Drawing for the job (mm, zero at the part's lowest x, y, z). A direction names the side the tool comes from. Give positions to 0.01 mm unless a question says otherwise; leave off trailing zeros. Loops run counter-clockwise (first coordinate to the right, second up) from the corner with the lowest first, then second, coordinate; pieces in that order, holes last.
1) Band-saw the part on B-B on x = 5. List the corners of the cut face in (y, z).
2) Two-plate mould, pull along Y, no slides. Class the marked faces 1, 2 and 3: +Y half, -Y half, draft (parallel to the pull), parting line (faces both ways), or undercut.
3) 3-axis set-ups, long thin cutter, end or side, ignore diameter. For the marked faces 4 and 5: which of +Z, -Z, +X, -X, +Y, -Y reach the whole face in a straight line?
4) Band-saw the part on A-A on z = 5.5. State how many separate pieces and enclosed holes the cut face has, then the cut area to 3 significant figures.
5) Wall check: line 1 (X direction, y = 3.5, z = 5.1) (1 decimal); line 2 (X direction, y = 10.5, z = 4.2) (1 decimal); line 3 (Y direction, x = 3.75, z = 4.5) (1 decimal). Give the ranges that are in metal, low to high.
6) Flat gauge pins, fed straight in: P1, Ø0.9, axis at x = 9.67, y = 6.25, coming from the -Z side; P2, Ø1, axis at x = 9.5, z = 2, coming from the +Y side; P3, Ø1.4, axis at x = 3.8, y = 9.59, coming from the +Z side. Where does each tip first touch, or does it go through?
7) Band-saw the part on D-D on z = 3.55. List the corners of the cut face in (x, y), then the cut area to 3 significant figures.
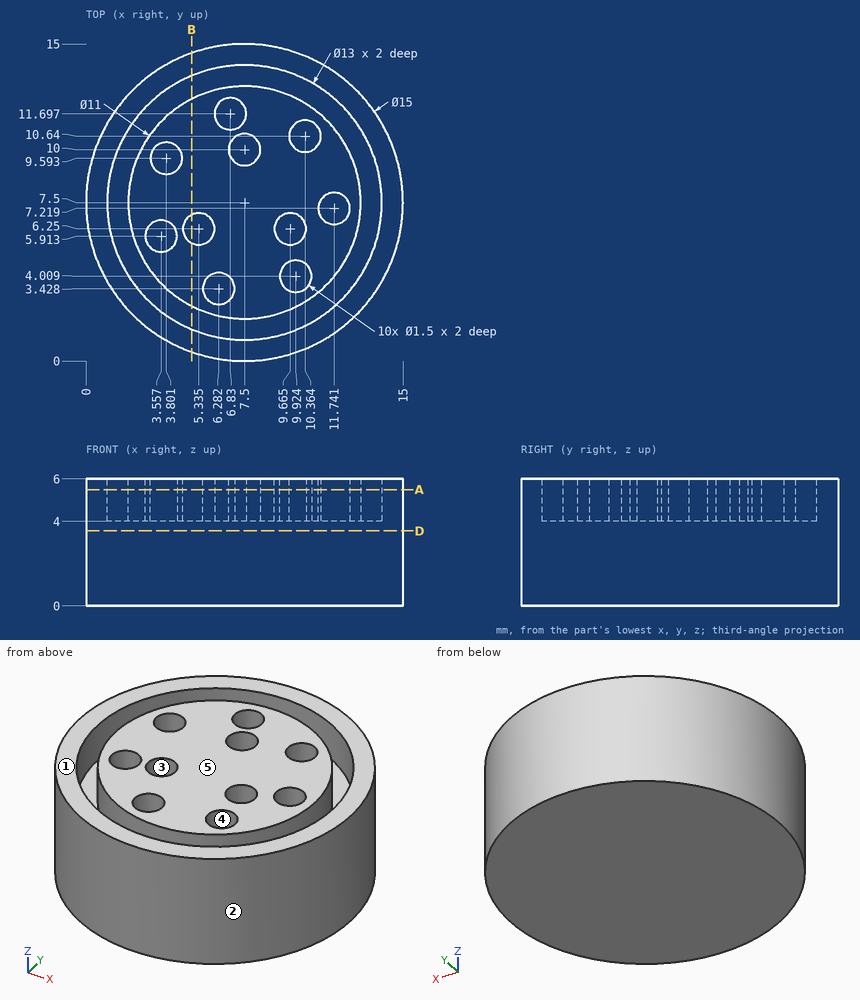
Findings below:
1. outline: (0.43, 0) - (14.57, 0) - (14.57, 6) - (13.5, 6) - (13.5, 4) - (12.4, 4) - (12.4, 6) - (6.92, 6) - (6.92, 4) - (5.58, 4) - (5.58, 6) - (2.6, 6) - (2.6, 4) - (1.5, 4) - (1.5, 6) - (0.43, 6) - close
2. face 1: draft
2. face 2: parting line
2. face 3: undercut
3. face 4: +Z
3. face 5: +Z, +X, -X, +Y, -Y
4. separate pieces: 2
4. enclosed holes: 11
4. area: 121 mm2
5. line 1: x = 1.2 to 2.4, 3.7 to 5.5, 7 to 9.4, 10.5 to 11.3, 12.6 to 13.8
5. line 2: x = 0.6 to 1.7, 2.9 to 6.9, 8.1 to 9.6, 11.1 to 12.1, 13.3 to 14.4
5. line 3: y = 1 to 2.2, 3.5 to 5.2, 6.6 to 8.8, 10.3 to 11.5, 12.8 to 14
6. P1: stops at z = 0
6. P2: stops at y = 14.85
6. P3: stops at z = 4
7. outline: circle Ø15 at (7.5, 7.5)
7. area: 177 mm2
